Input: dimensioned drawing with shaded views. Units: mm. Origin: part minimum x, y, z. A direction names the side the tool comes from. Give positions to 0.01 mm unless a question says otherwise; leave off trailing zeros. Order: outer loops, then holes, each group sorted by start corner. A loop starts at its lowest first (then second) coordinate and runs counter-clockwise, first axis right, second up.
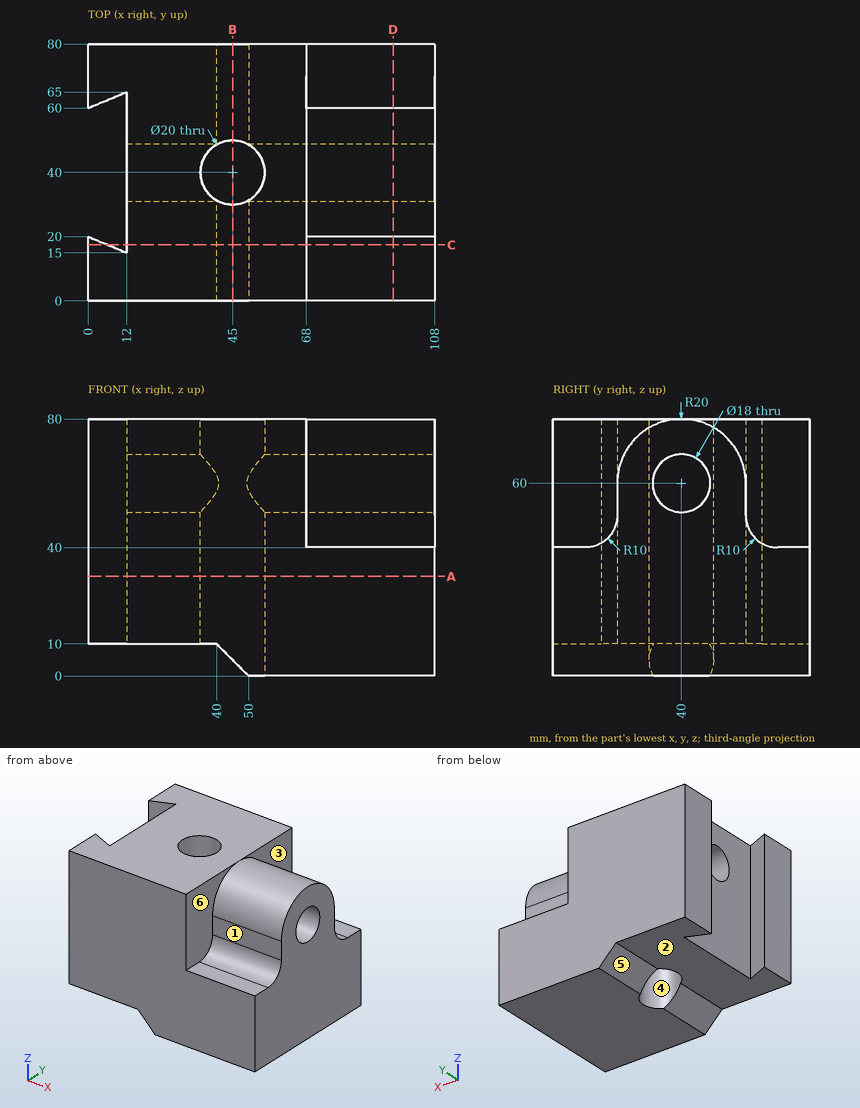
1) Section query B-B, the plane x = 45. Return the cut outline in (y, z), and give its area (3 significant figures).
Report:
outline: (0, 5) - (30, 5) - (30, 80) - (0, 80) - close; (50, 5) - (80, 5) - (80, 80) - (50, 80) - close
area: 4,500 mm2
2) Section query D-D, the plane x = 95. Return the cut outline in (y, z).
Report:
outline: (0, 0) - (80, 0) - (80, 40) - (70, 40) arc R10 cw to (60, 50) - (60, 60) arc R20 ccw to (20, 60) - (20, 50) arc R10 cw to (10, 40) - (0, 40) - close; hole circle Ø18 at (40, 60)
3) Reachability of the marked faces 1, 2 and 3 from +Z, -Z, +X, -X, +Y, -Y: full face, straight path, thin tool, end or side. Return the list, or none.
Report:
face 1: +Z, +X, -Y
face 2: -Z, -X, +Y, -Y
face 3: +Z, +X, +Y
4) Pin query (flat end, axial travel): pin 1 (1.5 mm diameter, centred on x = 48.5, z = 13.5, fed in from -Y); pin 2 (1.5 mm diameter, centred on x = 78, y = 69, fed in from +Z); pin 3 (4 mm diameter, centred on y = 24.5, z = 13.5, fed in from -X); pin 4 (3 mm diameter, centred on x = 81, z = 55, fed in from +Y). Return the tip coordinate at first contact, or that it passes through.
Report:
pin 1: stops at y = 0
pin 2: stops at z = 40.15
pin 3: stops at x = 12
pin 4: stops at y = 60
5) Section query C-C, the plane y = 17.5. Return the cut outline in (x, z).
Report:
outline: (0, 10) - (6, 10) - (6, 80) - (0, 80) - close; (12, 10) - (40, 10) - (50, 0) - (108, 0) - (108, 43.39) - (68, 43.39) - (68, 80) - (12, 80) - close
6) Draft query along X for the marked faces 4, 5 and 6. Return one class per face: +X half, -X half, draft (parallel to the pull), parting line (faces both ways), or undercut.
Report:
face 4: undercut
face 5: -X half
face 6: +X half
7) Section query A-A, the plane z = 31. Return the cut outline in (x, y), and give its area (3 significant figures).
Report:
outline: (0, 0) - (108, 0) - (108, 80) - (0, 80) - (0, 60) - (12, 65) - (12, 15) - (0, 20) - close; hole circle Ø20 at (45, 40)
area: 7,790 mm2
8) Material intervals for L1, parallel to Z at x = 53, y = 47.5; L2, parallel to Y at x = 45, z = 19.5; L3, parallel to X at y = 22, z = 47.5, sorted ascending.
Report:
L1: z = 0 to 55.03, 64.97 to 80
L2: y = 0 to 30, 50 to 80
L3: x = 12 to 108
